Geometry: final body of the model. Coordinates: model frame, mm. Coordinates: 2 decimals unless noted, no trailing zeros. Order: outer loops, then holes, each group sorted by start corner. A loop starts at its lowest first (then second) coordinate and runs counter-clockwise, first axis right, second up. Notation, with made-up numbers: M 45.5,-28.75 L 64.5,-28.75 A25 ccw 64.5,7.25 Z; hole C 32,-9 d1. An arc over 180 degrees is marked long. Write item = value, one per line.
Autodesk Inventor part; units mm, degrees
ref_plane "YZ Plane" through (0, 0, 0) normal (1, 0, 0) x (0, 1, 0)
ref_plane "XY Plane" through (0, 0, 0) normal (0, 0, 1) x (1, 0, 0)
sketch "Sketch1" plane through (0, 0, 0) normal (0, 0, 1) x (1, 0, 0)
  line L0 (0, 0) -> (12.7, 0)
  line L1 (12.7, 0) -> (12.7, 1.7272)
  line L2 (12.7, 1.7272) -> (0, 1.7272)
  line L3 (0, 1.7272) -> (0, 0)
  line L4 (0, -1.27) -> (12.7, -1.27)
  line L5 (12.7, -1.27) -> (12.7, -2.9972)
  line L6 (12.7, -2.9972) -> (0, -2.9972)
  line L7 (0, -2.9972) -> (0, -1.27)
  dimension "d0" = 12.7
  dimension "d1" = 1.7272
  dimension "d2" = 12.7
  dimension "d3" = 1.7272
  dimension "d4" = 1.27
ref_plane "Work Plane1" through (0, -0.635, 0) normal (0, 1, 0) x (-1, 0, 0)
sketch "Sketch2" plane through (0, -0.635, 0) normal (0, 1, 0) x (-1, 0, 0)
  line L0 (0, 23.6728) -> (-12.7, 23.6728)
  line L1 (-12.7, 23.6728) -> (-12.7, 25.4)
  line L2 (-12.7, 25.4) -> (0, 25.4)
  line L3 (0, 25.4) -> (0, 23.6728)
  point P0 (0, 0)
  point P1 (0, 24.5364)
  dimension "d6" = 12.7
  dimension "d7" = 1.7272
  dimension "d10" = 25.4
extrude "Extrusion1" add sketch "Sketch1" along normal blind 25.4
extrude "Extrusion2" add sketch "Sketch2" along normal blind 1.27 and the other way blind 1.27
properties part number "ClipConnector"
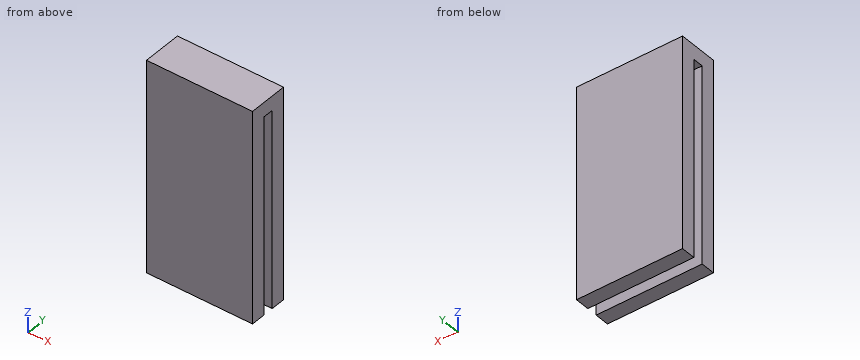
1) Section B-B, the plane x = 9.25. Return loops of the section in (y, z).
Numbers:
outline = M -3,0 L -1.27,0 L -1.27,23.67 L 0,23.67 L 0,0 L 1.73,0 L 1.73,25.4 L -3,25.4 Z
2) Line query: L1, parallel to Y at x = 6.5, z = 6.5; L2, parallel to Z at x = 6.5, y = -0.75. Output: solid intervals per line, ascending.
Numbers:
L1 = -3 to -1.27, 0 to 1.73
L2 = 23.67 to 25.4
3) Section A-A, the plane z = 1.75. Return loops of the section in (x, y), and give its area (3 significant figures).
Numbers:
outline = M 0,-3 L 12.7,-3 L 12.7,-1.27 L 0,-1.27 Z; M 0,0 L 12.7,0 L 12.7,1.73 L 0,1.73 Z
area = 43.9 mm²
4) Section C-C, the plane y = -1. Return loops of the section in (x, z).
Numbers:
outline = M 0,23.67 L 12.7,23.67 L 12.7,25.4 L 0,25.4 Z
